```python
from build123d import *

# Parameters (mm, degrees)
SKETCH1_R           = 6.35
SKETCH1_R_2         = 1.5875
BOSS_EXTRUDE1_DEPTH = 88.9
CUT_EXTRUDE1_DEPTH  = 89.9


with BuildPart() as part:
    # Sketch1 → Boss-Extrude1 (new body)
    with BuildSketch(Plane(origin=(0, 0, 0), x_dir=(1, 0, 0), z_dir=(0, 1, 0))):
        Circle(SKETCH1_R)
        Circle(SKETCH1_R_2, mode=Mode.SUBTRACT)
    extrude(amount=BOSS_EXTRUDE1_DEPTH)

    # Sketch2 → Cut-Extrude1 (cut, through all)
    with BuildSketch(Plane(origin=(0, 88.9, 0), x_dir=(1, 0, 0), z_dir=(0, 1, 0))):
        with BuildLine():
            ThreePointArc((-4.7625, 4.200130206), (-6.35, 0), (-4.7625, -4.200130206))
            Line((-4.7625, -4.200130206), (-4.7625, 4.200130206))
        make_face()
        with BuildLine():
            Line((4.7625, 4.200130206), (4.7625, -4.200130206))
            ThreePointArc((4.7625, -4.200130206), (5.939881102, -2.24506403), (6.35, 0))
            ThreePointArc((6.35, 0), (5.939881102, 2.24506403), (4.7625, 4.200130206))
        make_face()
    extrude(amount=-CUT_EXTRUDE1_DEPTH, mode=Mode.SUBTRACT)


solid = part.part
```
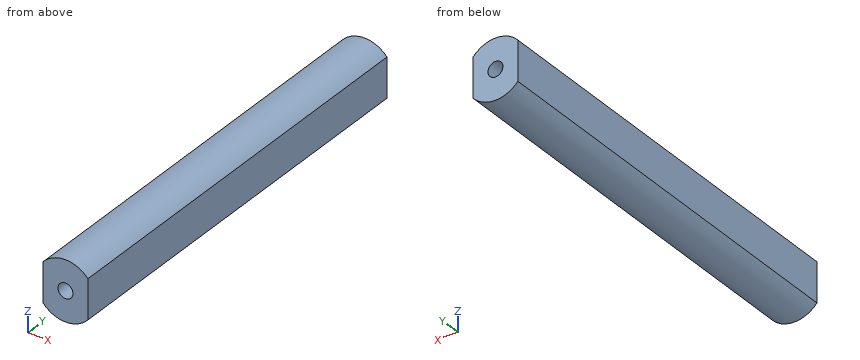
CAD build for the part. Positions are in the model's coordinates, mm. Give positions to 0.01 mm unless a question says otherwise; leave off trailing zeros. Loops run counter-clockwise (first coordinate to the right, second up) from the corner with the lowest first, then second, coordinate; pieces in that order, holes last. Notation, with made-up numbers: (59, -20) - (97, -20) arc R7 ccw to (97, -13) - close; hole circle Ø4 at (2, -27.5). An arc over 180 degrees is marked (long way). Put each result on its own line as item: value.
Q1. Slice it at A-A (z = 0). Give the cut face in (x, y), plus the area to 3 significant figures.
Filled in:
outline: (-4.76, 0) - (-1.59, 0) - (-1.59, 88.9) - (-4.76, 88.9) - close; (1.59, 0) - (4.76, 0) - (4.76, 88.9) - (1.59, 88.9) - close
area: 565 mm²
Q2. Slice it at C-C (x = 0). Give the cut face in (y, z).
Filled in:
outline: (0, -6.35) - (88.9, -6.35) - (88.9, -1.59) - (0, -1.59) - close; (0, 1.59) - (88.9, 1.59) - (88.9, 6.35) - (0, 6.35) - close
Q3. Probe line 1 along Z through (x, y) = (0, 62.5); line 2 along X through (y, z) = (66.5, 0); line 3 along Z through (x, y) = (1, 74). List the from-to ranges inside material, lowest first.
Filled in:
line 1: z = -6.35 to -1.59, 1.59 to 6.35
line 2: x = -4.76 to -1.59, 1.59 to 4.76
line 3: z = -6.27 to -1.23, 1.23 to 6.27
Q4. Slice it at D-D (x = 4). Give the cut face in (y, z).
Filled in:
outline: (0, -4.93) - (88.9, -4.93) - (88.9, 4.93) - (0, 4.93) - close
Q5. Flat gauge pins, fed straight in: pin 1 (3 mm diameter, centred on x = 0, z = 0, fed in from +Y); pin 2 (1.5 mm diameter, centred on x = 2.5, z = -4, fed in from -Y); pin 3 (1 mm diameter, centred on x = 1.5, y = 72, fed in from -Z). Where does each tip first touch, or does it go through?
Filled in:
pin 1: passes through
pin 2: stops at y = 0
pin 3: stops at z = -6.27
